Check sheet for the modelled part. Datum: model origin and axes. Units: mm. A direction names the side the tool comes from. Give positions to 0.01 mm unless a question says otherwise; leave off trailing zeros. Write each loop counter-clockwise with the first axis right and the second up, starting at its lowest first coordinate (ties: lowest second). Pieces come first, ordered by that corner, then holes. Notation, with made-up numbers: (0, 60.25) -> (59, 60.25) arc R8 ccw to (59, 73.25) -> close; hole circle Ø6 at (-14, -39). An arc over 180 degrees is marked (long way). Return JSON: item names as keys, results as strings.
from build123d import *

# Parameters (mm, degrees)
ESQUISSE1_W             = 170
ESQUISSE1_H             = 300
BOSS_EXTRU_1_DEPTH      = 15
ESQUISSE2_R             = 2.5
ENL_V_MAT_EXTRU_1_DEPTH = 15
ESQUISSE3_W             = 60
ESQUISSE3_H             = 25
ENL_V_MAT_EXTRU_2_DEPTH = 3
ESQUISSE4_R             = 3
ENL_V_MAT_EXTRU_3_DEPTH = 12
ENL_V_START             = -15
ESQUISSE5_R             = 2.5
ENL_V_MAT_EXTRU_4_DEPTH = 15
ESQUISSE6_R             = 3
ENL_V_MAT_EXTRU_5_DEPTH = 15


with BuildPart() as part:
    # Esquisse1 → Boss.-Extru.1 (new body)
    with BuildSketch(Plane.XY):
        with Locations((85, 150)):
            Rectangle(ESQUISSE1_W, ESQUISSE1_H)
    extrude(amount=BOSS_EXTRU_1_DEPTH)

    # Esquisse2 → Enlèv. mat.-Extru.1 (cut)
    with BuildSketch(Plane.XY.offset(15)):
        with Locations((9, 250)):
            Circle(ESQUISSE2_R)
        with Locations(Location((33, 250, 0), (0, 0, 180))):
            Circle(ESQUISSE2_R)
        with Locations((9, 150)):
            Circle(ESQUISSE2_R)
        with Locations(Location((33, 150, 0), (0, 0, 180))):
            Circle(ESQUISSE2_R)
        with Locations((33, 50)):
            Circle(ESQUISSE2_R)
        with Locations(Location((9, 50, 0), (0, 0, 180))):
            Circle(ESQUISSE2_R)
        with Locations((161, 50)):
            Circle(ESQUISSE2_R)
        with Locations(Location((137, 50, 0), (0, 0, 180))):
            Circle(ESQUISSE2_R)
        with Locations((137, 150)):
            Circle(ESQUISSE2_R)
        with Locations(Location((161, 150, 0), (0, 0, 180))):
            Circle(ESQUISSE2_R)
        with Locations((137, 250)):
            Circle(ESQUISSE2_R)
        with Locations(Location((161, 250, 0), (0, 0, 180))):
            Circle(ESQUISSE2_R)
    extrude(amount=-ENL_V_MAT_EXTRU_1_DEPTH, mode=Mode.SUBTRACT)

    # Esquisse3 → Enlèv. mat.-Extru.2 (cut)
    with BuildSketch(Plane(origin=(0, 0, 0), x_dir=(-1, 0, 0), z_dir=(0, 0, -1))):
        with Locations((-85, 287.5)):
            Rectangle(ESQUISSE3_W, ESQUISSE3_H)
    extrude(amount=-ENL_V_MAT_EXTRU_2_DEPTH, mode=Mode.SUBTRACT)

    # Esquisse4 → Enlèv. mat.-Extru.3 (cut)
    with BuildSketch(Plane(origin=(0, 0, 3), x_dir=(-1, 0, 0), z_dir=(0, 0, -1))):
        with Locations((-108, 293.5)):
            Circle(ESQUISSE4_R)
        with Locations((-62, 293.5)):
            Circle(ESQUISSE4_R)
        with Locations((-108, 282.5)):
            Circle(ESQUISSE4_R)
        with Locations((-62, 282.5)):
            Circle(ESQUISSE4_R)
    extrude(amount=-ENL_V_MAT_EXTRU_3_DEPTH, mode=Mode.SUBTRACT)

    # Esquisse5 → Enlèv. mat.-Extru.4 (cut)
    with BuildSketch(Plane.XY.offset(15).offset(ENL_V_START)):
        with Locations((47.5, 292.5)):
            Circle(ESQUISSE5_R)
        with Locations((47.5, 277.5)):
            Circle(ESQUISSE5_R)
        with Locations(Location((47.5, 262.5, 0), (0, 0, 180))):
            Circle(ESQUISSE5_R)
        with Locations((122.5, 262.5)):
            Circle(ESQUISSE5_R)
        with Locations(Location((122.5, 277.5, 0), (0, 0, 180))):
            Circle(ESQUISSE5_R)
        with Locations(Location((122.5, 292.5, 0), (0, 0, 180))):
            Circle(ESQUISSE5_R)
    extrude(amount=ENL_V_MAT_EXTRU_4_DEPTH, mode=Mode.SUBTRACT)

    # Esquisse6 → Enlèv. mat.-Extru.5 (cut)
    with BuildSketch(Plane.XY.offset(15)):
        with Locations((20, 100)):
            Circle(ESQUISSE6_R)
        with Locations((20, 125)):
            Circle(ESQUISSE6_R)
        with Locations(Location((20, 75, 0), (0, 0, 180))):
            Circle(ESQUISSE6_R)
        with Locations((150, 75)):
            Circle(ESQUISSE6_R)
        with Locations(Location((150, 125, 0), (0, 0, 180))):
            Circle(ESQUISSE6_R)
        with Locations(Location((150, 100, 0), (0, 0, 180))):
            Circle(ESQUISSE6_R)
    extrude(amount=-ENL_V_MAT_EXTRU_5_DEPTH, mode=Mode.SUBTRACT)


solid = part.part
(1) Set-up check for faces 1 (the flat face through (84, 152, 15)), 2 (the flat face through (85, 288, 3)): record each of +Z, -Z, +X, -X, +Y, -Y from which the full face is reachable in a straight line by a thin tool's end or side.
Reply:
{"face 1": "+Z, +X, -X, +Y, -Y", "face 2": "-Z, +Y"}
(2) Cross-section at C-C on x = 62. Enter the section's corners in (y, z), then the cut area to 3 significant figures.
Reply:
{"outline": "(0, 0) -> (275, 0) -> (275, 3) -> (279.5, 3) -> (279.5, 15) -> (0, 15) -> close; (285.5, 3) -> (290.5, 3) -> (290.5, 15) -> (285.5, 15) -> close; (296.5, 3) -> (300, 3) -> (300, 15) -> (296.5, 15) -> close", "area": "4,280 mm^2"}
(3) Release check for a two-part mould opening along X. For faces 3 (the flat face through (84, 300, 7)), 4 (the flat face through (0, 148, 7)), 5 (the cylindrical face through (148.616, 102.662, 7.605)) record: pulls with the +X half, pulls with the -X half, needs draft (parallel to the pull), parting line crosses it, or undercut.
Reply:
{"face 3": "needs draft", "face 4": "pulls with the -X half", "face 5": "undercut"}
(4) Cross-section at B-B on y = 125. Enter the section's corners in (x, z), then the cut area to 3 significant figures.
Reply:
{"outline": "(0, 0) -> (17, 0) -> (17, 15) -> (0, 15) -> close; (23, 0) -> (147, 0) -> (147, 15) -> (23, 15) -> close; (153, 0) -> (170, 0) -> (170, 15) -> (153, 15) -> close", "area": "2,370 mm^2"}
(5) Thickness scan on L1, parallel to Y at x = 33, z = 12; L2, parallel to Y at x = 20, z = 4.25; L3, parallel to Y at x = 108, z = 11.5. Record the ranges inside material, lowest first.
Reply:
{"L1": "0 to 47.5, 52.5 to 147.5, 152.5 to 247.5, 252.5 to 300", "L2": "0 to 72, 78 to 97, 103 to 122, 128 to 300", "L3": "0 to 279.5, 285.5 to 290.5, 296.5 to 300"}
(6) Cross-section at A-A on x = 20. Enter the section's corners in (y, z).
Reply:
{"outline": "(0, 0) -> (72, 0) -> (72, 15) -> (0, 15) -> close; (78, 0) -> (97, 0) -> (97, 15) -> (78, 15) -> close; (103, 0) -> (122, 0) -> (122, 15) -> (103, 15) -> close; (128, 0) -> (300, 0) -> (300, 15) -> (128, 15) -> close"}
